The figure shows three views and two pictorial views of one solid part (mm, origin at its lowest corner). Answer the questions. A direction names the side the tool comes from. Coordinates: 2 decimals unless noted, no trailing zeros. Order: outer loops, then holes, each group sorted by start corner. A loop starts at its lowest first (then second) coordinate and runs counter-clockwise, first axis right, second up. Notation, with made-up numbers: (15.5, 21.25) -> (71.5, 21.25) arc R21 cw to (71.5, 49.25) -> close; hole circle Ø1 at (-18.75, -29.75). An arc over 180 degrees is marked (long way). Write item = value, one per line. Start each with the question number.
Q1. The part is cut by section D-D, the plane y = 8.75. Determine the outline of the cut face in (x, z).
Q2. Straight lines are drawn through the part: L1, parallel to Z at x = 16, y = 6.25; L2, parallel to Y at x = 30, z = 12.75; L3, parallel to X at y = 7.5, z = 11.25 (1 decimal). For each, find the intervals that lie inside material, in ascending order. Write a range as from..to.
Q3. The part is cut by section C-C, the plane z = 12.25. Determine the outline of the cut face in (x, y), plus the area to 3 significant figures.
Q4. The part is cut by section A-A, the plane x = 16. Determine the outline of the cut face in (y, z).
Q5. Which of the six approach directions +Z, -Z, +X, -X, +Y, -Y give full straight-line access (tool end or side, diameter ignored) to the marked faces 1, 2 and 3?
Q6. Flat-ended cylindrical pins translate along their axes: pin 1 (2 mm diameter, centred on x = 2.5, z = 12, fed in from +Y); pin 2 (1.5 mm diameter, centred on y = 11.5, z = 14.5, fed in from +X). Find the tip coordinate at first contact, or state that the pin passes through.
Q7. The part is cut by section B-B, the plane z = 2.25. Determine the outline of the cut face in (x, y), plus the area to 3 significant figures.
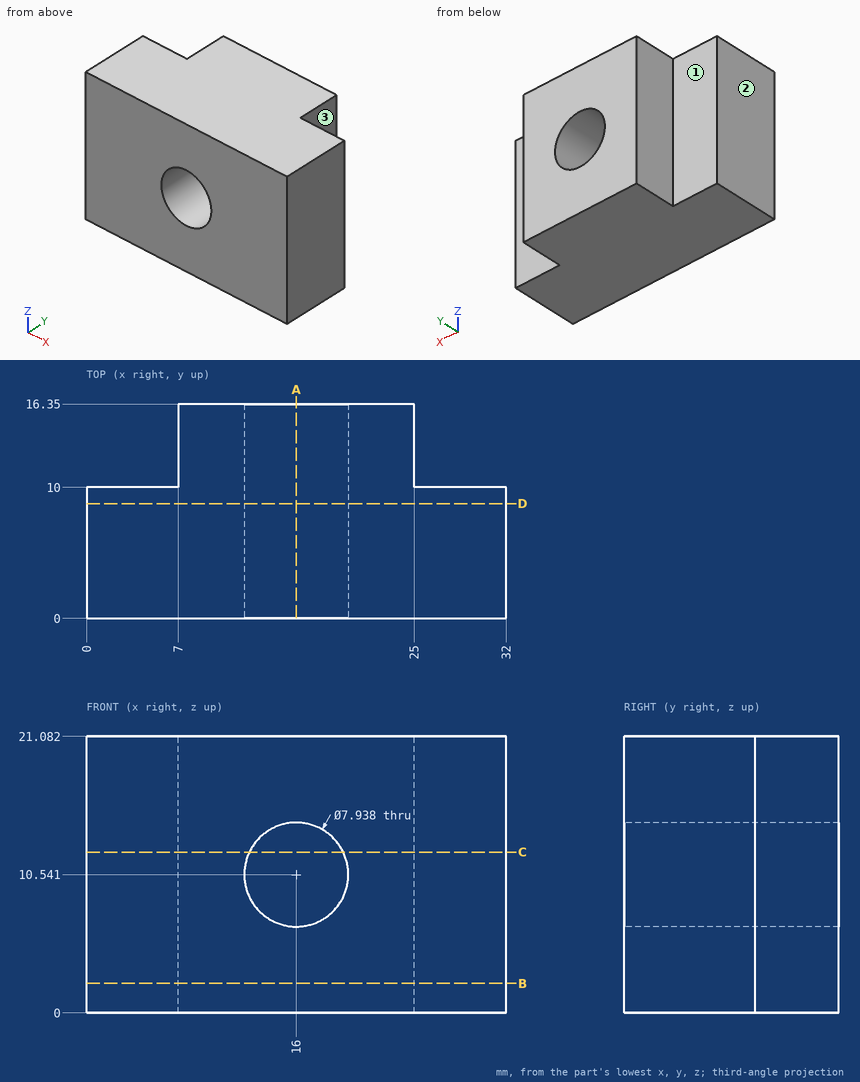
Model answer:
q1.outline = (0, 0) -> (32, 0) -> (32, 21.08) -> (0, 21.08) -> close; hole circle Ø7.94 at (16, 10.54)
q2.L1 = 0..6.57, 14.51..21.08
q2.L2 = 0..10
q2.L3 = 0..12.1, 19.9..32
q3.outline = (0, 0) -> (12.42, 0) -> (12.42, 16.35) -> (7, 16.35) -> (7, 10) -> (0, 10) -> close; (19.58, 0) -> (32, 0) -> (32, 10) -> (25, 10) -> (25, 16.35) -> (19.58, 16.35) -> close
q3.area = 317 mm2
q4.outline = (0, 0) -> (16.35, 0) -> (16.35, 6.57) -> (0, 6.57) -> close; (0, 14.51) -> (16.35, 14.51) -> (16.35, 21.08) -> (0, 21.08) -> close
q5.face_1 = +Z, -Z, -X, +Y
q5.face_2 = +Z, -Z, -X, +Y, -Y
q5.face_3 = +Z, -Z, +X, +Y
q6.pin_1 = 10
q6.pin_2 = 25
q7.outline = (0, 0) -> (32, 0) -> (32, 10) -> (25, 10) -> (25, 16.35) -> (7, 16.35) -> (7, 10) -> (0, 10) -> close
q7.area = 434 mm2
